Work out the finished part from the listing and answer in its coordinate system (mm). Face numbers are marked on the shaded views. Round coordinates to 2 decimals unless told otherwise and drop trailing zeros. Write each loop counter-clockwise with the first axis right and the second up, starting at its lowest first coordinate (ties: lowest second). Pieces come first, ordered by that corner, then holes. Notation, with made-up numbers: M 5.5,-11.5 L 38.5,-11.5 A16 ccw 38.5,-1.5 Z; hole C -7,27.25 d7. An arc over 180 degrees is marked long. Answer in a Markdown table with one row per item.
```python
from build123d import *

# Parameters (mm, degrees)
BOSS_EXTRUDE1_DEPTH = 1.5
SKETCH2_R           = 2.75
BOSS_EXTRUDE2_DEPTH = 6
SKETCH3_W           = 1.1
SKETCH3_H           = 1.45
SKETCH3_W_2         = 1.45
SKETCH3_H_2         = 1.1
SKETCH3_W_3         = 4
SKETCH3_H_3         = 4
CUT_EXTRUDE1_DEPTH  = 6
CHAMFER1_SIZE       = 0.3
FILLET1_R           = 1
FILLET3_R           = 0.2


with BuildPart() as part:
    # Sketch1 → Boss-Extrude1 (new body)
    with BuildSketch(Plane(origin=(0, 0, 0), x_dir=(1, 0, 0), z_dir=(0, 1, 0))):
        with BuildLine():
            Line((-109.324675649, 4.396717546), (4.675324351, 4.396717546))
            ThreePointArc((4.675324351, 4.396717546), (5.382431132, 4.103824327), (5.675324351, 3.396717546))
            Line((5.675324351, 3.396717546), (5.675324351, -8.603282454))
            ThreePointArc((5.675324351, -8.603282454), (5.382431132, -9.310389235), (4.675324351, -9.603282454))
            Line((4.675324351, -9.603282454), (-109.324675649, -9.603282454))
            ThreePointArc((-109.324675649, -9.603282454), (-110.03178243, -9.310389235), (-110.324675649, -8.603282454))
            Line((-110.324675649, -8.603282454), (-110.324675649, 3.396717546))
            ThreePointArc((-110.324675649, 3.396717546), (-110.03178243, 4.103824327), (-109.324675649, 4.396717546))
        make_face()
    extrude(amount=BOSS_EXTRUDE1_DEPTH)

    # Sketch2 → Boss-Extrude2 (add)
    with BuildSketch(Plane.XZ):
        with Locations(Location((-52.324675649, 2.603282454, 0), (0, 0, 90))):
            Circle(SKETCH2_R)
        with Locations(Location((-102.324675649, 2.603282454, 0), (0, 0, 90))):
            Circle(SKETCH2_R)
        with Locations(Location((-2.324675649, 2.603282454, 0), (0, 0, 90))):
            Circle(SKETCH2_R)
    extrude(amount=BOSS_EXTRUDE2_DEPTH)

    # Sketch3 → Cut-Extrude1 (cut)
    with BuildSketch(Plane.XZ.offset(6)):
        with Locations((-52.324675649, 3.878282454)):
            Rectangle(SKETCH3_W, SKETCH3_H)
        with Locations((-51.049675649, 2.603282454)):
            Rectangle(SKETCH3_W_2, SKETCH3_H_2)
        with Locations((-52.324675649, 2.603282454)):
            Rectangle(SKETCH3_W, SKETCH3_H_2)
        with Locations((-53.599675649, 2.603282454)):
            Rectangle(SKETCH3_W_2, SKETCH3_H_2)
        with Locations((-52.324675649, 1.328282454)):
            Rectangle(SKETCH3_W, SKETCH3_H)
        with Locations((-2.53698339, 2.603282454)):
            Rectangle(SKETCH3_W_3, SKETCH3_H_2)
        with Locations((-2.53698339, 2.603282454)):
            Rectangle(SKETCH3_W, SKETCH3_H_3)
        with Locations((-102.324675649, 2.603282454)):
            Rectangle(SKETCH3_W, SKETCH3_H_3)
        with Locations((-102.324675649, 2.603282454)):
            Rectangle(SKETCH3_W_3, SKETCH3_H_2)
    extrude(amount=-CUT_EXTRUDE1_DEPTH, mode=Mode.SUBTRACT)

    # Chamfer1
    chamfer1_edges = [part.edges().sort_by_distance(p)[0] for p in [
        (-1.26198339, -6, 2.053282454),
        (-3.08698339, -6, 3.878282454),
        (-4.53698339, -6, 2.603282454),
        (-3.81198339, -6, 2.053282454),
        (-3.08698339, -6, 1.328282454),
        (-2.53698339, -6, 0.603282454),
        (-3.81198339, -6, 3.153282454),
        (-0.53698339, -6, 2.603282454),
        (-1.26198339, -6, 3.153282454),
        (-2.53698339, -6, 4.603282454),
        (-1.98698339, -6, 3.878282454),
        (-1.98698339, -6, 1.328282454),
        (-103.599675649, -6, 2.053282454),
        (-102.874675649, -6, 1.328282454),
        (-102.324675649, -6, 0.603282454),
        (-101.049675649, -6, 2.053282454),
        (-102.874675649, -6, 3.878282454),
        (-104.324675649, -6, 2.603282454),
        (-102.324675649, -6, 4.603282454),
        (-101.774675649, -6, 3.878282454),
        (-101.774675649, -6, 1.328282454),
        (-100.324675649, -6, 2.603282454),
        (-101.049675649, -6, 3.153282454),
        (-103.599675649, -6, 3.153282454),
        (-51.774675649, -6, 3.878282454),
        (-51.049675649, -6, 3.153282454),
        (-50.324675649, -6, 2.603282454),
        (-51.774675649, -6, 1.328282454),
        (-53.599675649, -6, 3.153282454),
        (-52.324675649, -6, 4.603282454),
        (-52.874675649, -6, 3.878282454),
        (-54.324675649, -6, 2.603282454),
        (-53.599675649, -6, 2.053282454),
        (-52.874675649, -6, 1.328282454),
        (-52.324675649, -6, 0.603282454),
        (-51.049675649, -6, 2.053282454),
    ]]
    chamfer(chamfer1_edges, length=CHAMFER1_SIZE)

    # Fillet1
    fillet1_edges = [part.edges().sort_by_distance(p)[0] for p in [
        (-52.324675649, 0, -0.146717546),
        (-102.324675649, 0, -0.146717546),
        (-2.324675649, 0, -0.146717546),
    ]]
    fillet(fillet1_edges, radius=FILLET1_R)

    # Fillet3
    fillet3_edges = [part.edges().sort_by_distance(p)[0] for p in [
        (5.382431132, 1.5, 9.310389235),
        (-52.324675649, 0, 9.603282454),
        (-110.03178243, 0, 9.310389235),
        (5.675324351, 1.5, 2.603282454),
        (5.382431132, 1.5, -4.103824327),
        (-52.324675649, 1.5, -4.396717546),
        (-110.03178243, 1.5, -4.103824327),
        (-110.324675649, 1.5, 2.603282454),
        (-110.03178243, 1.5, 9.310389235),
        (-52.324675649, 1.5, 9.603282454),
        (-110.324675649, 0, 2.603282454),
        (-110.03178243, 0, -4.103824327),
        (-52.324675649, 0, -4.396717546),
        (5.382431132, 0, -4.103824327),
        (5.675324351, 0, 2.603282454),
        (5.382431132, 0, 9.310389235),
    ]]
    fillet(fillet3_edges, radius=FILLET3_R)


solid = part.part
```
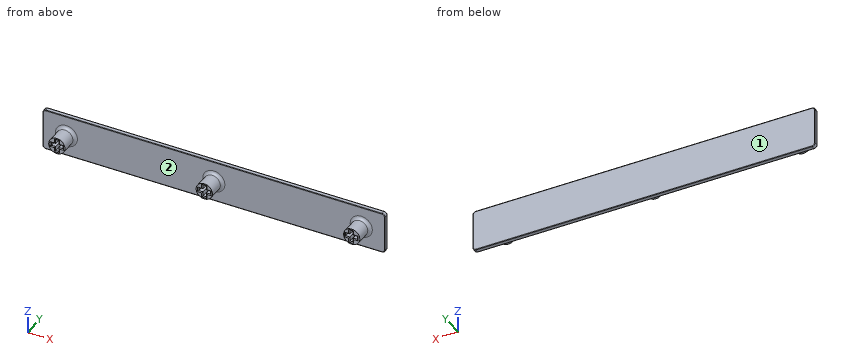
1. Determine the mould class of the marked faces 1 and 2 for opening direction X: released by +X, released by -X, zero draft, split by the parting line, or undercut.
Calculated:
| item | result |
|---|---|
| face 1 | zero draft |
| face 2 | undercut |
2. The part is cut by section C-C (y = -4.75). Count the separate pieces of the cut face and the enclosed holes in it, plus the area to 3 significant figures.
Calculated:
| item | result |
|---|---|
| separate pieces | 3 |
| enclosed holes | 3 |
| area | 48.5 mm² |
3. The part is cut by section B-B (z = -2.25). Determine the outline of the cut face in (x, y).
Calculated:
| item | result |
|---|---|
| outline | M -110.32,0.2 A0.2 ccw -110.12,0 L 5.48,0 A0.2 ccw 5.68,0.2 L 5.68,1.3 A0.2 ccw 5.48,1.5 L -110.12,1.5 A0.2 ccw -110.32,1.3 Z |
4. Given pin 1 (4 mm diameter, centred on x = -82.5, z = 3, fed in from -Y); pin 2 (0.7 mm diameter, centred on y = -3, z = 4, fed in from +X); pin 3 (1.6 mm diameter, centred on x = -104, y = -3, fed in from -Z); pin 4 (1 mm diameter, centred on y = -4, z = -2, fed in from +X), each flat-ended and moving along its own axis, determine where each tip first touches the part or whether it passes through.
Calculated:
| item | result |
|---|---|
| pin 1 | stops at y = 0 |
| pin 2 | stops at x = 0.22 |
| pin 3 | stops at z = 0 |
| pin 4 | passes through |
5. Consider line 1 along X through (y, z) = (-4, 2); line 2 along X through (y, z) = (-1.75, 3.5); line 3 along X through (y, z) = (-1.5, 5). Determine where each line is inside the solid, lowest interval first. Write a range as from..to.
Calculated:
| item | result |
|---|---|
| line 1 | x = -105.01..-102.87, -101.77..-99.64, -55.01..-52.87, -51.77..-49.64, -5.01..-3.09, -1.99..0.36 |
| line 2 | x = -104.92..-102.87, -101.77..-99.72, -54.92..-52.87, -51.77..-49.72, -4.92..-3.09, -1.99..0.28 |
| line 3 | x = -103.67..-100.98, -53.67..-50.98, -3.67..-0.98 |
6. The part is cut by section A-A (x = -36). Determine the outline of the cut face in (y, z), plus the area to 3 significant figures.
Calculated:
| item | result |
|---|---|
| outline | M 0,-4.2 A0.2 ccw 0.2,-4.4 L 1.3,-4.4 A0.2 ccw 1.5,-4.2 L 1.5,9.4 A0.2 ccw 1.3,9.6 L 0.2,9.6 A0.2 ccw 0,9.4 Z |
| area | 21.0 mm² |
